Geometry: final body of the model. Coordinates: model frame, mm. A direction names the side the tool comes from. Round coordinates to 2 decimals unless told otherwise and drop trailing zeros. Loops run counter-clockwise (first coordinate to the right, second up) from the corner with the lowest first, then second, coordinate; pieces in that order, holes last. Notation, with made-up numbers: (38.25, -11) -> (46.25, -11) arc R16 ccw to (46.25, -6) -> close; hole circle Ø10 at (16, 28.5). An arc over 180 degrees is marked (long way). Answer in a Markdown table with one row per item.
Autodesk Inventor part; units mm, degrees
ref_plane "re_XY" through (0, 0, 0) normal (0, 1, 0) x (1, 0, 0)
ref_plane "re_YZ" through (0, 0, 0) normal (1, 0, 0) x (0, 0, -1)
ref_plane "re_ZX" through (0, 0, 0) normal (0, 0, -1) x (0, 1, 0)
sketch "Skizze_1" plane through (0, 0, 0) normal (0, 1, 0) x (-1, 0, 0)
  line L0 (35, -20) -> (35, 20)
  line L1 (35, 20) -> (0, 20)
  arc A0 (0, 20) -> (0, -20) centre (0, 0) ccw
  line L2 (0, -20) -> (35, -20)
extrude "Extrusion1" add sketch "Skizze_1" along normal mid plane 40
sketch "Skizze_2" plane through (0, 0, 0) normal (0, 0, 1) x (1, 0, 0)
  line L0 (-21, 20) -> (-21, 13)
  line L1 (-21, 13) -> (20, 13)
  line L2 (20, 13) -> (20, 20)
  line L3 (20, 20) -> (-21, 20)
extrude "Extrusion2" cut sketch "Skizze_2" along normal mid plane 40
sketch "Skizze_3" plane through (0, 0, 0) normal (0, 0, 1) x (1, 0, 0)
  line L0 (-21, -13) -> (20, -13)
  line L1 (20, -13) -> (20, 0.3)
  line L2 (20, 0.3) -> (-21, 0.3)
  line L3 (-21, 0.3) -> (-21, -13)
extrude "Extrusion3" cut sketch "Skizze_3" along normal mid plane 40
sketch "Skizze_4" plane through (20, 0, 0) normal (1, 0, 0) x (0, 0, -1)
  circle A0 centre (0, 0) radius 7.6
extrude "Extrusion4" cut sketch "Skizze_4" against normal blind 47.5
sketch "Sketch5" plane through (-35, -20, -20) normal (-1, 0, 0) x (0, 0, 1)
  point P0 (20, 20)
hole "Drilling 2" at (-35, 0, 0) direction (1, 0, 0) diameter 8.4 depth 11
sketch "Skizze_6" plane through (-35, 0, 0) normal (1, 0, 0) x (0, 0, -1)
  line L0 (-20, -6.1) -> (-6.1, -6.1)
  line L1 (-6.1, -6.1) -> (-6.1, -20)
  line L2 (-6.1, -20) -> (6.1, -20)
  line L3 (6.1, -20) -> (6.1, -6.1)
  line L4 (6.1, -6.1) -> (20, -6.1)
  line L5 (20, -6.1) -> (20, 6.1)
  line L6 (20, 6.1) -> (6.1, 6.1)
  line L7 (6.1, 6.1) -> (6.1, 20)
  line L8 (6.1, 20) -> (-6.1, 20)
  line L9 (-6.1, 20) -> (-6.1, 6.1)
  line L10 (-6.1, 6.1) -> (-20, 6.1)
  line L11 (-20, 6.1) -> (-20, -6.1)
extrude "Extrusion5" cut sketch "Skizze_6" along normal blind 3
sketch "Skizze_7" plane through (-35, 0, 0) normal (1, 0, 0) x (0, 0, -1)
  line L0 (18.2, 20) -> (20, 18.2)
  line L1 (20, 18.2) -> (20, 20)
  line L2 (20, 20) -> (18.2, 20)
extrude "Extrusion6" cut sketch "Skizze_7" along normal blind 55
sketch "Skizze_8" plane through (-35, 0, 0) normal (1, 0, 0) x (0, 0, -1)
  line L0 (-20, 20) -> (-20, 18.2)
  line L1 (-20, 18.2) -> (-18.2, 20)
  line L2 (-18.2, 20) -> (-20, 20)
extrude "Extrusion7" cut sketch "Skizze_8" along normal blind 55
sketch "Skizze_9" plane through (-35, 0, 0) normal (1, 0, 0) x (0, 0, -1)
  line L0 (-20, -20) -> (-18.2, -20)
  line L1 (-18.2, -20) -> (-20, -18.2)
  line L2 (-20, -18.2) -> (-20, -20)
extrude "Extrusion8" cut sketch "Skizze_9" along normal blind 55
sketch "Skizze_10" plane through (-35, 0, 0) normal (1, 0, 0) x (0, 0, -1)
  line L0 (18.2, -20) -> (20, -20)
  line L1 (20, -20) -> (20, -18.2)
  line L2 (20, -18.2) -> (18.2, -20)
extrude "Extrusion9" cut sketch "Skizze_10" along normal blind 55
sketch "Sketch11" plane through (0, -20, 0) normal (0, -1, 0) x (1, 0, 0)
  point P0 (0, 0)
hole "Drilling 3" at (0, -20, 0) direction (0, 1, 0) diameter 10 depth 40
sketch "Skizze_12" plane through (0, -20, 0) normal (0, 1, 0) x (1, 0, 0)
  circle A0 centre (0, 0) radius 8.4
extrude "Extrusion10" cut sketch "Skizze_12" along normal blind 4
sketch "Skizze_13" plane through (0, 0, 20) normal (0, 0, 1) x (1, 0, 0)
  circle A0 centre (0, 7) radius 3.3235
extrude "Extrusion11" cut sketch "Skizze_13" against normal blind 20
ref_plane "re_XY" through (0, 0, 0) normal (0, 1, 0) x (1, 0, 0)
ref_plane "re_YZ" through (0, 0, 0) normal (1, 0, 0) x (0, 0, -1)
ref_plane "re_ZX" through (0, 0, 0) normal (0, 0, -1) x (0, 1, 0)
ref_plane "bo1_XY" through (0, -20, 0) normal (0, 1, 0) x (1, 0, 0)
ref_plane "bo1_YZ" through (0, -20, 0) normal (1, 0, 0) x (0, 0, -1)
ref_plane "bo1_ZX" through (0, -20, 0) normal (0, 0, -1) x (0, 1, 0)
ref_plane "hebel_XY" through (0, 16, 0) normal (0, 1, 0) x (1, 0, 0)
ref_plane "hebel_YZ" through (0, 16, 0) normal (1, 0, 0) x (0, 0, -1)
ref_plane "hebel_ZX" through (0, 16, 0) normal (0, 0, -1) x (0, 1, 0)
properties part number "May Tec 1.63.14041_Base plates"
Item 1: Reachability of faces 1 (the face through (-34, 13, -6.1)), 2 (the face through (-34, -6.1, 13)), 3 (the face through (4, -16, 4)), 4 (the face through (-8.695, 7.535, 0.989)), 5 (the face through (-1, 0.3, -14)) from +Z, -Z, +X, -X, +Y, -Y: full face, straight path, thin tool, end or side. Return the list, or none.
Answer:
| item | result |
|---|---|
| face 1 | -X, +Y, -Y |
| face 2 | +Z, -Z, -X |
| face 3 | -Y |
| face 4 | +X |
| face 5 | +Z, -Z, +X |
Item 2: Cut plane A-A (x = -13). Output: boundary loops of the cut face in (y, z).
Answer:
| item | result |
|---|---|
| outline | (-20, -18.2) -> (-18.2, -20) -> (-13, -20) -> (-13, 20) -> (-18.2, 20) -> (-20, 18.2) -> close; (0.3, -20) -> (13, -20) -> (13, 20) -> (0.3, 20) -> (0.3, 7.59) arc R7.6 cw to (0.3, -7.59) -> close |
Item 3: Line query: probe 1 along Z at (x, y) = (-28.75, 0); probe 2 along Y at (x, z) = (5, -14.5); probe 3 along X at (y, z) = (-19.1, 0). Output: solid intervals per line, ascending. Write a range as [from, to].
Answer:
| item | result |
|---|---|
| probe 1 | z = [-20, -4.2], [4.2, 20] |
| probe 2 | y = [-20, -13], [0.3, 13] |
| probe 3 | x = [-32, -8.4], [8.4, 20] |
Item 4: Cut plane C-C (y = 17.5). Output: boundary loops of the cut face in (x, z), then the cut area to 3 significant figures.
Answer:
| item | result |
|---|---|
| outline | (-35, -20) -> (-21, -20) -> (-21, 20) -> (-35, 20) -> (-35, 6.1) -> (-32, 6.1) -> (-32, -6.1) -> (-35, -6.1) -> close |
| area | 523 mm² |
Item 5: Cut plane D-D (x = -1). Output: boundary loops of the cut face in (y, z).
Answer:
| item | result |
|---|---|
| outline | (-20, -18.2) -> (-18.2, -20) -> (-13, -20) -> (-13, -4.9) -> (-16, -4.9) -> (-16, -8.34) -> (-20, -8.34) -> close; (-20, 8.34) -> (-16, 8.34) -> (-16, 4.9) -> (-13, 4.9) -> (-13, 20) -> (-18.2, 20) -> (-20, 18.2) -> close; (0.3, -20) -> (13, -20) -> (13, -4.9) -> (5.81, -4.9) arc R7.6 cw to (0.3, -7.59) -> close; (0.3, 7.59) arc R7.6 cw to (3.83, 6.56) -> (3.83, 20) -> (0.3, 20) -> close; (10.17, 4.9) -> (13, 4.9) -> (13, 20) -> (10.17, 20) -> close |
Item 6: Draft query along X for faces 6 (the face through (4.88, -14.48, 1.08)), 7 (the face through (-1, 0.3, 14)), 8 (the face through (-35, -13, 13)). Return one class per face: pulls with the +X half, pulls with the -X half, needs draft (parallel to the pull), parting line crosses it, or undercut.
Answer:
| item | result |
|---|---|
| face 6 | undercut |
| face 7 | needs draft |
| face 8 | pulls with the -X half |
Item 7: Pin query (flat end, axial travel): pin 1 Ø20 at (x, z) = (8.5, 5.5) entering from +Y; pin 2 Ø5 at (x, y) = (2.5, 6.5) entering from +Z; pin 3 Ø16 at (x, z) = (0, 0) entering from -Y; pin 4 Ø3 at (x, z) = (-1, -2.5) entering from +Y. Return the tip coordinate at first contact, or that it passes through.
Answer:
| item | result |
|---|---|
| pin 1 | stops at y = 13 |
| pin 2 | stops at z = 19.93 |
| pin 3 | stops at y = -16 |
| pin 4 | passes through |
Item 8: Cut plane B-B (z = 0). Output: boundary loops of the cut face in (x, y).
Answer:
| item | result |
|---|---|
| outline | (-32, -20) -> (-8.4, -20) -> (-8.4, -16) -> (-5, -16) -> (-5, -13) -> (-21, -13) -> (-21, -7.6) -> (-27.5, -7.6) -> (-27.5, -4.2) -> (-32, -4.2) -> close; (-32, 4.2) -> (-27.5, 4.2) -> (-27.5, 7.6) -> (-5, 7.6) -> (-5, 13) -> (-21, 13) -> (-21, 20) -> (-32, 20) -> close; (5, -16) -> (8.4, -16) -> (8.4, -20) -> (20, -20) -> (20, -13) -> (5, -13) -> close; (5, 7.6) -> (20, 7.6) -> (20, 13) -> (5, 13) -> close |
